from build123d import *

# Parameters (mm, degrees)
SKETCH1_R           = 65
BOSS_EXTRUDE2_DEPTH = 25
SKETCH2_R           = 60
CUT_EXTRUDE1_DEPTH  = 20
SKETCH3_W           = 40
SKETCH3_H           = 50
BOSS_EXTRUDE3_DEPTH = 20
SKETCH4_W           = 35
SKETCH4_H           = 28
CUT_EXTRUDE2_DEPTH  = 18


with BuildPart() as part:
    # Sketch1 → Boss-Extrude2 (new body)
    with BuildSketch(Plane(origin=(0, 0, 0), x_dir=(1, 0, 0), z_dir=(0, 1, 0))):
        with Locations(Location((0, 0, 0), (0, 0, 270))):
            Circle(SKETCH1_R)
    extrude(amount=BOSS_EXTRUDE2_DEPTH)

    # Sketch2 → Cut-Extrude1 (cut)
    with BuildSketch(Plane(origin=(0, 25, 0), x_dir=(1, 0, 0), z_dir=(0, 1, 0))):
        with Locations(Location((0, 0, 0), (0, 0, 270))):
            Circle(SKETCH2_R)
    extrude(amount=-CUT_EXTRUDE1_DEPTH, mode=Mode.SUBTRACT)

    # Sketch3 → Boss-Extrude3 (add)
    with BuildSketch(Plane(origin=(0, 5, 0), x_dir=(1, 0, 0), z_dir=(0, 1, 0))):
        Rectangle(SKETCH3_W, SKETCH3_H)
    extrude(amount=BOSS_EXTRUDE3_DEPTH)

    # Sketch4 → Cut-Extrude2 (cut)
    with BuildSketch(Plane.XZ):
        with Locations((0, 9)):
            Rectangle(SKETCH4_W, SKETCH4_H)
    extrude(amount=-CUT_EXTRUDE2_DEPTH, mode=Mode.SUBTRACT)


solid = part.part
Geometry check sheet. Reference: the model listing, model coordinates, mm. A direction names the side the tool comes from. Coordinates: 2 decimals unless noted, no trailing zeros. Write each loop counter-clockwise with the first axis right and the second up, starting at its lowest first coordinate (ties: lowest second). Pieces come first, ordered by that corner, then holes. Notation, with made-up numbers: (63.5, -30) -> (76.5, -30) arc R27 ccw to (76.5, -11) -> close; hole circle Ø3 at (37, 75). An arc over 180 degrees is marked (long way). One line per question, with ' | ' between items.
1. Draft check along Z on faces 4 (the flat face through (0, 15, 25)), 5 (the cylindrical face through (19.52, 12.32, 62)), 6 (the flat face through (1, 0, -15)). Enter one of: +Z half, -Z half, draft (parallel to the pull), parting line (faces both ways), or undercut.
Answers:
face 4: undercut | face 5: parting line | face 6: draft
2. Cross-section at B-B on y = 6.5. Record the cut outline in (x, z).
Answers:
outline: circle Ø130 at (0, 0); (-20, -25) -> (20, -25) -> (20, 25) -> (-20, 25) -> close; hole circle Ø120 at (0, 0); hole (-17.5, -5) -> (17.5, -5) -> (17.5, 23) -> (-17.5, 23) -> close
3. Depth check by flat-ended pin: pin 1 Ø9 at (x, y) = (-0.5, 13) entering from +Z; pin 2 Ø2 at (y, z) = (12.5, 17.5) entering from +X; pin 3 Ø8 at (y, z) = (6, -12.5) entering from -X; pin 4 Ø3 at (x, y) = (14, 3) entering from -Z. Enter the tip coordinate at first touch or a pass-through.
Answers:
pin 1: stops at z = 65 | pin 2: stops at x = 62.87 | pin 3: stops at x = -64.44 | pin 4: stops at z = -63.79
4. Cross-section at D-D on z = 0. Record the cut outline in (x, y), and give its area (3 significant figures).
Answers:
outline: (-65, 0) -> (-17.5, 0) -> (-17.5, 18) -> (17.5, 18) -> (17.5, 0) -> (65, 0) -> (65, 25) -> (60, 25) -> (60, 5) -> (20, 5) -> (20, 25) -> (-20, 25) -> (-20, 5) -> (-60, 5) -> (-60, 25) -> (-65, 25) -> close | area: 1,020 mm²
5. Thickness scan on probe 1 along X at (y, z) = (13.25, 0); probe 2 along X at (y, z) = (18.5, 0); probe 3 along X at (y, z) = (22.5, -23.5). Record the ranges inside material, lowest first. Write a range as from..to.
Answers:
probe 1: x = -65..-60, -20..-17.5, 17.5..20, 60..65 | probe 2: x = -65..-60, -20..20, 60..65 | probe 3: x = -60.6..-55.21, -20..20, 55.21..60.6
6. Cross-section at C-C on x = 0. Record the cut outline in (y, z).
Answers:
outline: (0, -65) -> (25, -65) -> (25, -60) -> (5, -60) -> (5, -25) -> (25, -25) -> (25, 25) -> (5, 25) -> (5, 60) -> (25, 60) -> (25, 65) -> (0, 65) -> (0, 23) -> (18, 23) -> (18, -5) -> (0, -5) -> close
7. Cross-section at A-A on y = 22. Record the cut outline in (x, z), and give its area (3 significant figures).
Answers:
outline: circle Ø130 at (0, 0); (-20, -25) -> (20, -25) -> (20, 25) -> (-20, 25) -> close; hole circle Ø120 at (0, 0) | area: 3,960 mm²
8. Set-up check for faces 1 (the flat face through (-17.5, 9, 9)), 2 (the flat face through (0, 25, 0)), 3 (the cylindrical face through (2.64, 15.14, -59.94)): record each of +Z, -Z, +X, -X, +Y, -Y from which the full face is reachable in a straight line by a thin tool's end or side.
Answers:
face 1: -Y | face 2: +Z, -Z, +X, -X, +Y | face 3: +Y
